Geometry: final body of the model. Coordinates: model frame, mm. Round coordinates to 2 decimals unless told otherwise and drop trailing zeros. Order: outer loops, then holes, each group sorted by start corner. A loop starts at its lowest first (then second) coordinate and runs counter-clockwise, first axis right, second up. Notation, with made-up numbers: (80, -23) - (106, -23) arc R29 cw to (106, 12) - close; hole circle Ø2 at (78.25, -26.75). An arc over 180 degrees is marked (long way). Put each result on its own line as item: value. Start each with the question number.
(1) Material intervals for L1, parallel to X at y = 1.15, z = -26.5; L2, parallel to Z at x = 5.1, y = 1.5, sorted ascending. Write a range as [from, to].
(2) Section A-A (z = -102.5). Output: boundary loops of the cut face in (x, y).
(3) Section B-B (x = 114.9). Output: boundary loops of the cut face in (y, z).
(4) Pin query (flat end, axial travel): P1, Ø5, axis at x = 5.1, z = -42.5, coming from the -Y side; P2, Ø4, axis at x = 114.9, z = -42.5, coming from the -Y side. Return the tip coordinate at first contact, or that it passes through.
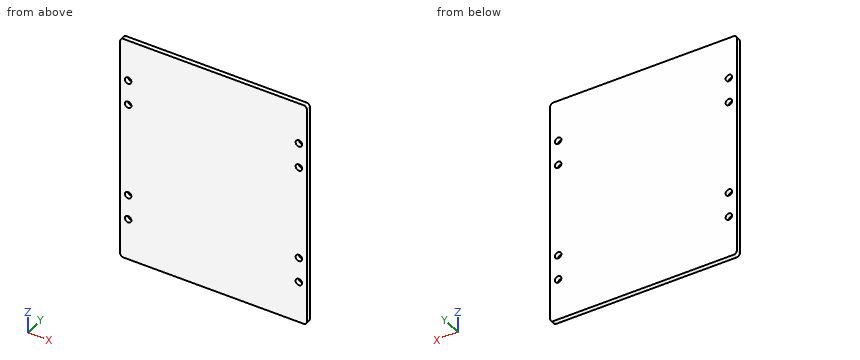
from build123d import *

# Parameters (mm, degrees)
SKETCH1_W           = 120
SKETCH1_H           = 145
BOSS_EXTRUDE1_DEPTH = 3
SKETCH2_R           = 2.1
CUT_EXTRUDE1_DEPTH  = 4
FILLET1_R           = 2


with BuildPart() as part:
    # Sketch1 → Boss-Extrude1 (new body)
    with BuildSketch(Plane(origin=(0, 0, 0), x_dir=(1, 0, 0), z_dir=(0, 1, 0))):
        with Locations((60, 72.5)):
            Rectangle(SKETCH1_W, SKETCH1_H)
    extrude(amount=BOSS_EXTRUDE1_DEPTH)

    # Sketch2 → Cut-Extrude1 (cut, through all)
    with BuildSketch(Plane(origin=(0, 3, 3), x_dir=(1, 0, 0), z_dir=(0, 1, 0))):
        with Locations((5.1, 121.5)):
            Circle(SKETCH2_R)
        with Locations((5.1, 105.5)):
            Circle(SKETCH2_R)
        with Locations((5.1, 45.5)):
            Circle(SKETCH2_R)
        with Locations((5.1, 29.5)):
            Circle(SKETCH2_R)
        with Locations((114.9, 29.5)):
            Circle(SKETCH2_R)
        with Locations((114.9, 45.5)):
            Circle(SKETCH2_R)
        with Locations((114.9, 105.5)):
            Circle(SKETCH2_R)
        with Locations((114.9, 121.5)):
            Circle(SKETCH2_R)
    extrude(amount=-CUT_EXTRUDE1_DEPTH, mode=Mode.SUBTRACT)

    # Fillet1
    fillet1_edges = [part.edges().sort_by_distance(p)[0] for p in [
        (0, 1.5, -145),
        (120, 1.5, -145),
        (120, 1.5, 0),
        (0, 1.5, 0),
    ]]
    fillet(fillet1_edges, radius=FILLET1_R)


solid = part.part
Checks:
1. L1: x = [0, 3], [7.2, 112.8], [117, 120]
1. L2: z = [-145, -120.6], [-116.4, -104.6], [-100.4, -44.6], [-40.4, -28.6], [-24.4, 0]
2. outline: (0, 0) - (3, 0) - (3, 3) - (0, 3) - close; (7.2, 0) - (112.8, 0) - (112.8, 3) - (7.2, 3) - close; (117, 0) - (120, 0) - (120, 3) - (117, 3) - close
3. outline: (0, -145) - (3, -145) - (3, -120.6) - (0, -120.6) - close; (0, -116.4) - (3, -116.4) - (3, -104.6) - (0, -104.6) - close; (0, -100.4) - (3, -100.4) - (3, -44.6) - (0, -44.6) - close; (0, -40.4) - (3, -40.4) - (3, -28.6) - (0, -28.6) - close; (0, -24.4) - (3, -24.4) - (3, 0) - (0, 0) - close
4. P1: stops at y = 0
4. P2: passes through
